The drawing under review shows one solid part. Ordinate dimensions are in mm from its lowest x, y, z. A direction names the side the tool comes from. Give positions to 0.01 mm unless a question says otherwise; leave off trailing zeros. Write each loop counter-clockwise with the first axis right and the second up, starting at its lowest first coordinate (ties: lowest second). Pieces come first, ordered by that corner, then holes. Notation, with made-up numbers: (22.5, -36) -> (79.5, -36) arc R28 cw to (79.5, -14) -> close; hole circle Ø11 at (53, 83.5). An arc over 180 degrees is marked (long way). Write item = value, one per line.
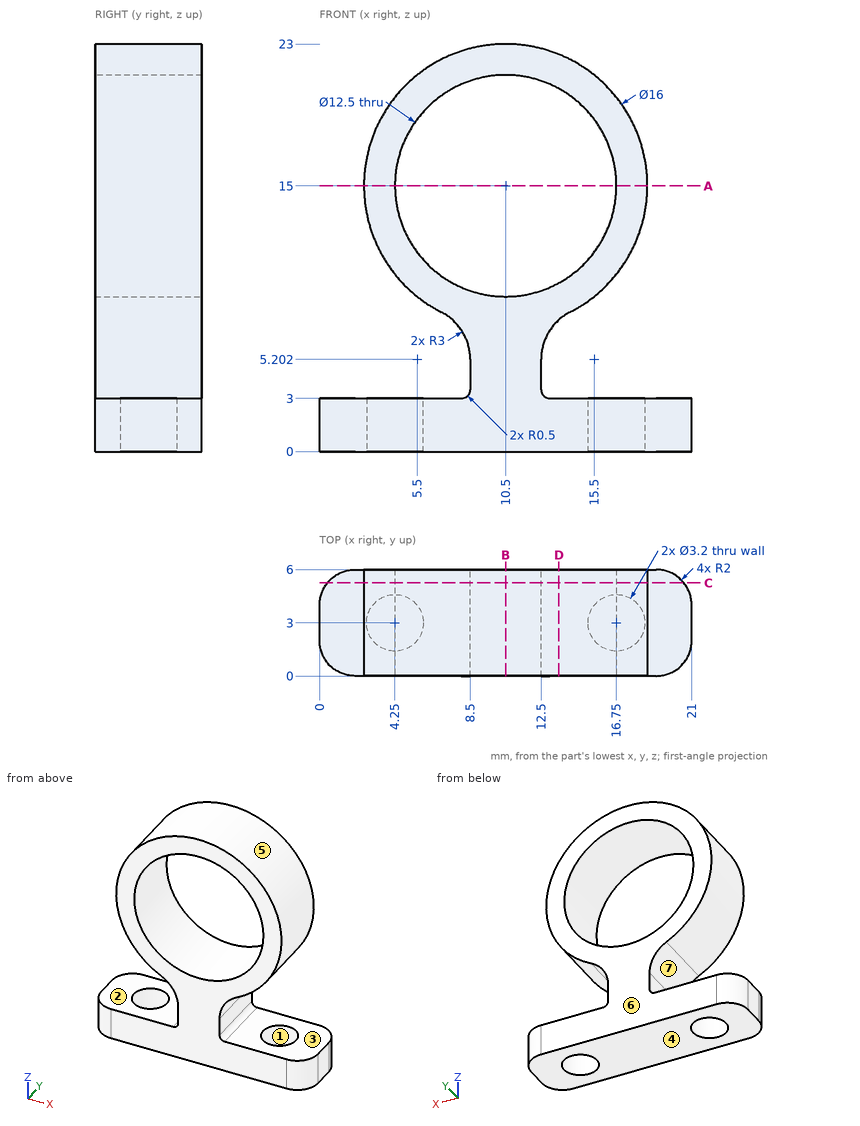
(1) Take a section at A-A (z = 15). Write out the cut boundary in (x, y).
Answers below:
outline = (2.5, 0) -> (4.25, 0) -> (4.25, 6) -> (2.5, 6) -> close; (16.75, 0) -> (18.5, 0) -> (18.5, 6) -> (16.75, 6) -> close
(2) Tool access review of the marked faces 1, 2 and 3: name each direction out of +Z, -Z, +X, -X, +Y, -Y from which nothing blocks a thin tool from reaching the whole face with its end or side.
Answers below:
face_1 = -Z
face_2 = -X, +Y, -Y
face_3 = +X, +Y, -Y
(3) To check wall thickness, follow probe 1 along Y at (x, z) = (4.25, 0.85); probe 2 along X at (y, z) = (4.25, 15); probe 3 along Z at (x, y) = (8.25, 3.5). State the ranges of each line that lie inside material, in increasing order.
Answers below:
probe_1 = 0 to 1.4, 4.6 to 6
probe_2 = 2.5 to 4.25, 16.75 to 18.5
probe_3 = 0 to 3.07, 6.4 to 9.17, 20.83 to 22.68
(4) The part is to be moulded in two halves that separate along Z. For the marked faces 4, 5, 6 and 7, say which applies: released by +Z, released by -Z, zero draft, split by the parting line, or undercut.
Answers below:
face_4 = released by -Z
face_5 = undercut
face_6 = zero draft
face_7 = undercut
(5) Take a section at B-B (x = 10.5). Write out the cut boundary in (y, z).
Answers below:
outline = (0, 0) -> (6, 0) -> (6, 8.75) -> (0, 8.75) -> close; (0, 21.25) -> (6, 21.25) -> (6, 23) -> (0, 23) -> close
(6) Take a section at C-C (y = 5.25). Write out the cut boundary in (x, z), plus the area to 3 significant figures.
Answers below:
outline = (0.44, 0) -> (20.56, 0) -> (20.56, 3) -> (13, 3) arc R0.5 cw to (12.5, 3.5) -> (12.5, 5.2) arc R3 cw to (14.14, 7.87) arc R8 ccw (long way) to (6.86, 7.87) arc R3 cw to (8.5, 5.2) -> (8.5, 3.5) arc R0.5 cw to (8, 3) -> (0.44, 3) -> close; hole circle Ø12.5 at (10.5, 15)
area = 157 mm^2
(7) For pin 1 (3 mm diameter, centred on x = 4.5, y = 3.5, fed in from +Z); pin 2 (1.9 mm diameter, centred on x = 16.75, y = 3, fed in from +Z); pin 3 (2 mm diameter, centred on y = 1.5, z = 19.5, fed in from +X), all flat-tipped, find the tip position at first contact; note any pin that passes through.
Answers below:
pin_1 = 21.61
pin_2 = 20.99
pin_3 = 17.69
(8) Take a section at D-D (x = 13.5). Write out the cut boundary in (y, z), plus the area to 3 significant figures.
Answers below:
outline = (0, 0) -> (6, 0) -> (6, 3) -> (0, 3) -> close; (0, 7.44) -> (6, 7.44) -> (6, 9.52) -> (0, 9.52) -> close; (0, 20.48) -> (6, 20.48) -> (6, 22.42) -> (0, 22.42) -> close
area = 42.1 mm^2
